Geometry check sheet. Reference: the model listing, model coordinates, mm. Face numbers are marked on the shaded views. A direction names the side the tool comes from. Give positions to 0.01 mm unless a question says otherwise; leave off trailing zeros. Order: outer loops, then holes, each group sorted by start corner. A loop starts at its lowest first (then second) coordinate and runs counter-clockwise, first axis right, second up. Notation, with made-up numbers: M 42,21.25 L 53,21.25 A19 ccw 53,39.25 Z; hole C 38,-24 d5. An arc over 180 degrees is marked long. One line per question, with ' | ' between items. Start each with the question number.
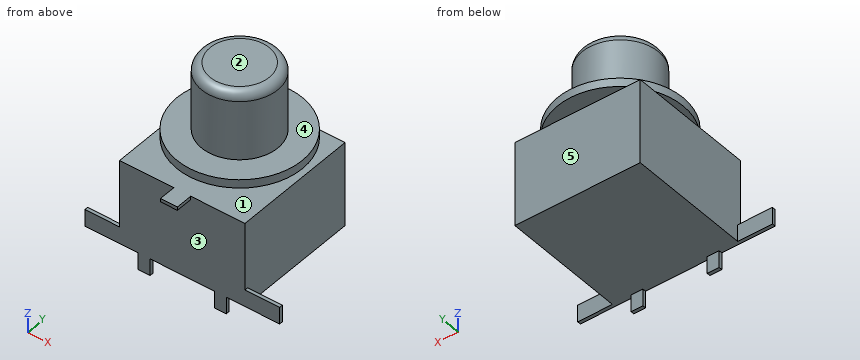
from build123d import *

# Parameters (mm, degrees)
SKETCH_1_W      = 7.4
SKETCH_1_H      = 7.5
EXTRUDE_1_DEPTH = 5
SKETCH_2_R      = 1.75
EXTRUDE_2_DEPTH = 2.2
FILLET_1_R      = 0.5
SKETCH_5_W      = 1
SKETCH_5_H      = 0.2
EXTRUDE_3_DEPTH = 2.05
SKETCH_6_W      = 1
SKETCH_6_H      = 0.2
EXTRUDE_4_DEPTH = 2.05
SKETCH_7_W      = 0.7
SKETCH_7_H      = 0.2
EXTRUDE_5_DEPTH = 1
SKETCH_8_W      = 1
SKETCH_8_H      = 0.2
EXTRUDE_6_DEPTH = 1


with BuildPart() as part:
    # 草图1 → 凸台-拉伸1 (new body)
    with BuildSketch(Plane.XY):
        Rectangle(SKETCH_1_W, SKETCH_1_H)
    extrude(amount=EXTRUDE_1_DEPTH)

    # 草图2 → 凸台-拉伸2 (add)
    with BuildSketch(Plane.XY.offset(5)):
        with Locations((0, 0.55)):
            Circle(SKETCH_2_R)
    extrude(amount=EXTRUDE_2_DEPTH)

    # 草图4 → 旋转1 (revolve)
    with BuildSketch(Plane(origin=(0, 0.55, 0), x_dir=(1, 0, 0), z_dir=(0, 1, 0)), mode=Mode.PRIVATE) as revolve_1_sk:
        Polygon((0, -5.5), (3.7, -5.5), (3.7, -6), (2.25, -6), (2.25, -10), (0, -10), align=None)
    revolve(revolve_1_sk.sketch.rotate(Axis((0, 0.55, -1.831178889), (0, 0, 1)), 180), axis=Axis((0, 0.55, -1.831178889), (0, 0, 1)))

    # 圆角1
    fillet_1_edges = [part.edges().sort_by_distance(p)[0] for p in [
        (2.25, 0.55, 10),
    ]]
    fillet(fillet_1_edges, radius=FILLET_1_R)

    # 草图5 → 凸台-拉伸3 (add)
    with BuildSketch(Plane(origin=(3.7, 0, 0), x_dir=(0, 0, -1), z_dir=(1, 0, 0))):
        with Locations((-0.5, -3.65)):
            Rectangle(SKETCH_5_W, SKETCH_5_H)
    extrude(amount=EXTRUDE_3_DEPTH)

    # 草图6 → 凸台-拉伸4 (add)
    with BuildSketch(Plane.ZY.offset(3.7)):
        with Locations((0.5, -3.65)):
            Rectangle(SKETCH_6_W, SKETCH_6_H)
    extrude(amount=EXTRUDE_4_DEPTH)

    # 草图7 → 凸台-拉伸5 (add)
    with BuildSketch(Plane(origin=(0, 0, 0), x_dir=(-1, 0, 0), z_dir=(0, 0, -1))):
        with Locations((-2.25, -3.65)):
            Rectangle(SKETCH_7_W, SKETCH_7_H)
        with Locations((2.25, -3.65)):
            Rectangle(SKETCH_7_W, SKETCH_7_H)
    extrude(amount=EXTRUDE_5_DEPTH)

    # 草图8 → 凸台-拉伸6 (add)
    with BuildSketch(Plane.XZ.offset(3.75)):
        with Locations((0, 4.9)):
            Rectangle(SKETCH_8_W, SKETCH_8_H)
    extrude(amount=EXTRUDE_6_DEPTH)


solid = part.part
Item 1: Set-up check for the marked faces 4 and 5: record each of +Z, -Z, +X, -X, +Y, -Y from which the full face is reachable in a straight line by a thin tool's end or side.
Item 2: Depth check by flat-ended pin: pin 1 (3 mm diameter, centred on x = -3.5, y = 2.5, fed in from +Z); pin 2 (1.5 mm diameter, centred on y = -1.5, z = 3.5, fed in from +X); pin 3 (1.1 mm diameter, centred on x = 5, z = 0.5, fed in from +Y). Enter the tip coordinate at first touch or a pass-through.
Item 3: Cross-section at D-D, the plane z = 2.25. Record the cut outline in (x, y), plus the area to 3 significant figures.
Item 4: Material ranges on line 1 along Z through (x, y) = (-2, 2); line 2 along Z through (x, y) = (0, 0); line 3 along X through (y, z) = (0, 4), recorded low to high.
Item 5: Cross-section at B-B, the plane y = 0.55. Record the cut outline in (x, z), plus the area to 3 significant figures.
Item 6: Cross-section at C-C, the plane x = 0. Record the cut outline in (y, z).
Item 7: Cross-section at A-A, the plane x = -3.5. Record the cut outline in (y, z), plus the area to 3 significant figures.
Item 8: Mould release check, pull along Z, two halves, no side actions. Record for the marked faces 1, 2 and 3: released by +Z, released by -Z, zero draft, split by the parting line, or undercut.
Outcome:
1) face 4: +Z | face 5: -Z, +X, -X, +Y
2) pin 1: stops at z = 6 | pin 2: stops at x = 3.7 | pin 3: stops at y = -3.55
3) outline: M -3.7,-3.75 L 3.7,-3.75 L 3.7,3.75 L -3.7,3.75 Z | area: 55.5 mm²
4) line 1: z = 0 to 5, 5.5 to 6 | line 2: z = 0 to 10 | line 3: x = -3.7 to 3.7
5) outline: M -3.7,0 L 3.7,0 L 3.7,5 L 1.75,5 L 1.75,5.5 L 3.7,5.5 L 3.7,6 L 2.25,6 L 2.25,9.5 A0.5 ccw 1.75,10 L -1.75,10 A0.5 ccw -2.25,9.5 L -2.25,6 L -3.7,6 L -3.7,5.5 L -1.75,5.5 L -1.75,5 L -3.7,5 Z | area: 60.3 mm²
6) outline: M -4.75,4.8 L -3.75,4.8 L -3.75,0 L 3.75,0 L 3.75,5 L 2.3,5 L 2.3,5.5 L 4.25,5.5 L 4.25,6 L 2.8,6 L 2.8,9.5 A0.5 ccw 2.3,10 L -1.2,10 A0.5 ccw -1.7,9.5 L -1.7,6 L -3.15,6 L -3.15,5.5 L -1.2,5.5 L -1.2,5 L -4.75,5 Z
7) outline: M -3.75,0 L 3.75,0 L 3.75,5 L -3.75,5 Z; M -0.65,5.5 L 1.75,5.5 L 1.75,6 L -0.65,6 Z | area: 38.7 mm²
8) face 1: undercut | face 2: released by +Z | face 3: zero draft
